Check sheet for the modelled part. Datum: model origin and axes. Units: mm. Face numbers are marked on the shaded views. A direction names the side the tool comes from. Round coordinates to 2 decimals unless told otherwise and drop trailing zeros. Write each loop counter-clockwise with the first axis right and the second up, starting at its lowest first coordinate (ties: lowest second). Pieces come first, ordered by that corner, then holes. Notation, with made-up numbers: (-16, -35.5) -> (-4, -35.5) arc R22 cw to (-4, -1.5) -> close; hole circle Ø5 at (34.25, 9.5). An arc over 180 degrees is marked (long way). Answer as a JSON object with one key per item and string values. Group by question number.
```python
from build123d import *

# Parameters (mm, degrees)
F3_DEPTH = 1.1
F4_SIZE  = 0.25


with BuildPart() as f1:
    # F0 (on Front) → F1 (revolve)
    with BuildSketch(Plane.XZ):
        Polygon((-1.6, -4.240741), (0, -4.240741), (0, 3.759259), (-2.95, 3.759259), (-1.6, 2.409259), align=None)
    revolve(axis=Axis((0, 0, -0.240741), (0, 0, -1)))

    # F2 (on face) → F3 (cut)
    with BuildSketch(Plane.XY.offset(3.759259)):
        Polygon((0.583124, -1.01), (1.166248, 0), (0.583124, 1.01), (-0.583124, 1.01), (-1.166248, 0), (-0.583124, -1.01), align=None)
    extrude(amount=-F3_DEPTH, mode=Mode.SUBTRACT)

    # F4
    f4_edges = [f1.edges().sort_by_distance(p)[0] for p in [
        (1.6, 0, -4.240741),
    ]]
    chamfer(f4_edges, length=F4_SIZE)


solid = f1.part
```
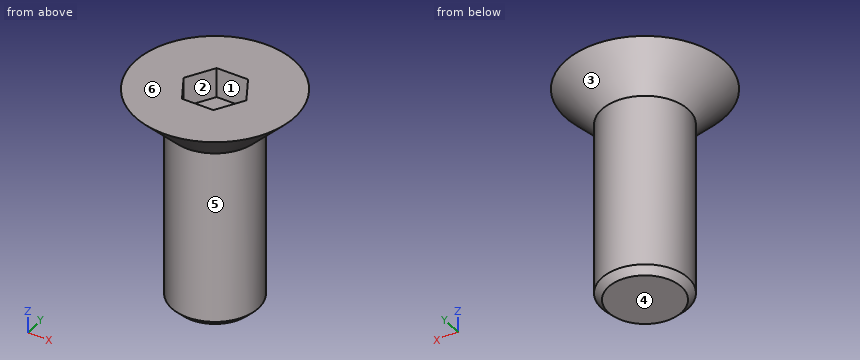
(1) Section check B-B on z = 1.5. Record the cut outline in (x, y).
(2) Scan lines: line 1 along Z through (x, y) = (-0.5, -0.7); line 2 along Y through (x, z) = (0, 2.25); line 3 along Z through (x, y) = (-1.45, 0.1). Record each from-to range of solid material in increasing order.
(3) Release check for a two-part mould opening along Y. For the marked faces 1, 2, 3 and 4 record: pulls with the +Y half, pulls with the -Y half, needs draft (parallel to the pull), parting line crosses it, or undercut.
(4) Section check A-A on x = 0. Record the cut outline in (y, z), then the cut area to 3 significant figures.
(5) Access from +Z, -Z, +X, -X, +Y, -Y to the whole of each face (thin tool, end or side, straight path). Record for the marked faces 5 and 6.
(6) Go/stop test with flat-tipped pins: pin 1 Ø3 at (y, z) = (-2, -2) entering from +X; pin 2 Ø1 at (y, z) = (0.5, 2) entering from +X; pin 3 Ø2 at (x, z) = (-0.5, 0.5) entering from +Y. Record where each tip stops, or that it passes through.
Data:
{
 "1": {"outline": "circle Ø3.2 at (0, 0)"},
 "2": {"line 1": "z = -4.24 to 2.66", "line 2": "y = -1.6 to 1.6", "line 3": "z = -4.14 to 3.76"},
 "3": {"face 1": "undercut", "face 2": "undercut", "face 3": "parting line crosses it", "face 4": "needs draft"},
 "4": {"outline": "(-2.95, 3.76) -> (-1.6, 2.41) -> (-1.6, -3.99) -> (-1.35, -4.24) -> (1.35, -4.24) -> (1.6, -3.99) -> (1.6, 2.41) -> (2.95, 3.76) -> (1.01, 3.76) -> (1.01, 2.66) -> (-1.01, 2.66) -> (-1.01, 3.76) -> close", "area": "25.1 mm²"},
 "5": {"face 5": "-Z", "face 6": "+Z, +X, -X, +Y, -Y"},
 "6": {"pin 1": "stops at x = 1.52", "pin 2": "stops at x = 1.63", "pin 3": "stops at y = 1.6"}
}
